Geometry check sheet. Reference: drawing and pictorial views, mm from the part's lowest x, y, z. A direction names the side the tool comes from. Round coordinates to 2 decimals unless told otherwise and drop trailing zeros. Write each loop counter-clockwise with the first axis right and the second up, starting at its lowest first coordinate (ties: lowest second). Pieces come first, ordered by that corner, then holes. Notation, with made-up numbers: (10.5, 41) -> (21.5, 41) arc R17 cw to (21.5, 66) -> close; hole circle Ø11 at (52.5, 24.25). An arc over 180 degrees is marked (long way). Write item = value, one per line.
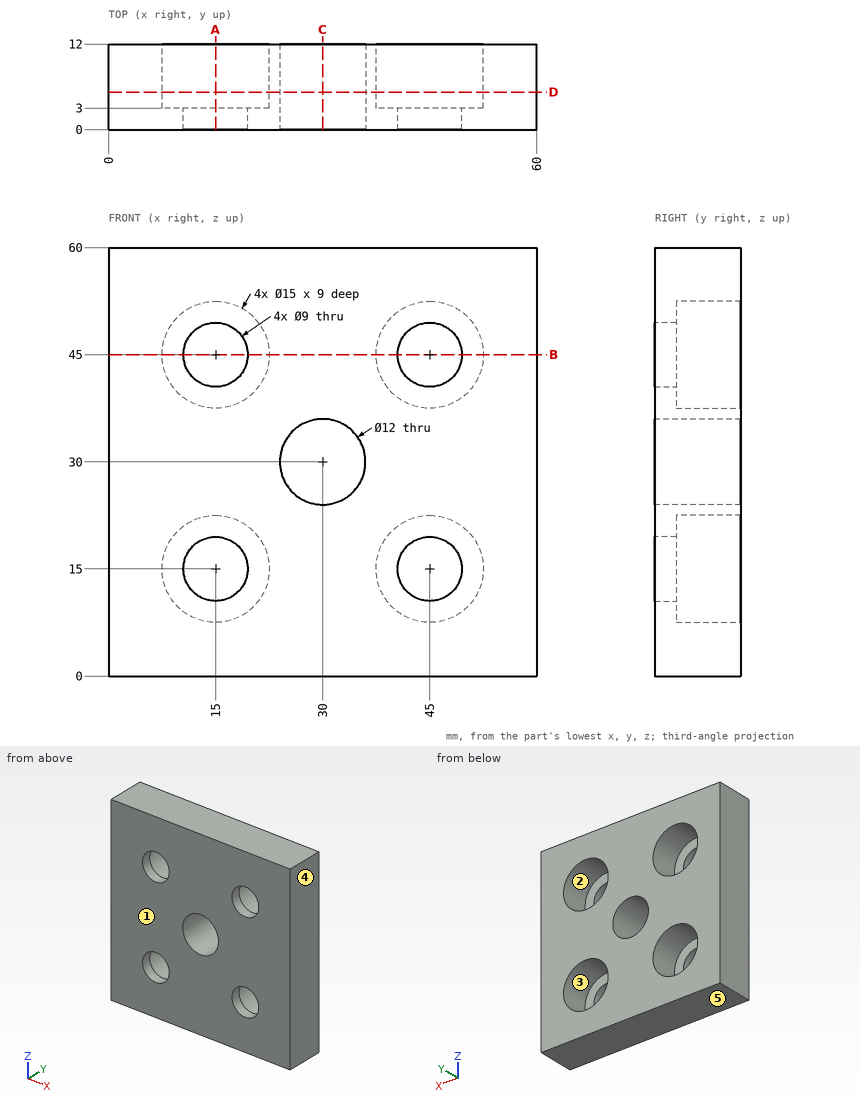
(1) Go/stop test with a flat-tipped pin: P1, Ø7.5, axis at x = 44, z = 48.5, coming from the +Y side. Record where the tip stops, or that it passes through.
Worked answers:
P1 = 3
(2) Sectioned sample at D-D on y = 5.25. Enter the section's corners in (x, z).
Worked answers:
outline = (0, 0) -> (60, 0) -> (60, 60) -> (0, 60) -> close; hole circle Ø15 at (15, 15); hole circle Ø15 at (15, 45); hole circle Ø12 at (30, 30); hole circle Ø15 at (45, 15); hole circle Ø15 at (45, 45)
(3) Sectioned sample at C-C on x = 30. Enter the section's corners in (y, z), then the cut area to 3 significant figures.
Worked answers:
outline = (0, 0) -> (12, 0) -> (12, 24) -> (0, 24) -> close; (0, 36) -> (12, 36) -> (12, 60) -> (0, 60) -> close
area = 576 mm²
(4) Release check for a two-part mould opening along Z. For the marked faces 3, 4 and 5 record: pulls with the +Z half, pulls with the -Z half, needs draft (parallel to the pull), parting line crosses it, or undercut.
Worked answers:
face_3 = undercut
face_4 = needs draft
face_5 = pulls with the -Z half
(5) Sectioned sample at B-B on z = 45. Enter the section's corners in (x, y).
Worked answers:
outline = (0, 0) -> (10.5, 0) -> (10.5, 3) -> (7.5, 3) -> (7.5, 12) -> (0, 12) -> close; (19.5, 0) -> (40.5, 0) -> (40.5, 3) -> (37.5, 3) -> (37.5, 12) -> (22.5, 12) -> (22.5, 3) -> (19.5, 3) -> close; (49.5, 0) -> (60, 0) -> (60, 12) -> (52.5, 12) -> (52.5, 3) -> (49.5, 3) -> close
(6) Material ranges on L1, parallel to X at y = 1.8, z = 15; L2, parallel to Z at x = 14.5, y = 7; L3, parallel to X at y = 8, z = 45, recorded low to high. Write a range as [from, to].
Worked answers:
L1 = [0, 10.5], [19.5, 40.5], [49.5, 60]
L2 = [0, 7.52], [22.48, 37.52], [52.48, 60]
L3 = [0, 7.5], [22.5, 37.5], [52.5, 60]
(7) Sectioned sample at A-A on x = 15. Enter the section's corners in (y, z), then the cut area to 3 significant figures.
Worked answers:
outline = (0, 0) -> (12, 0) -> (12, 7.5) -> (3, 7.5) -> (3, 10.5) -> (0, 10.5) -> close; (0, 19.5) -> (3, 19.5) -> (3, 22.5) -> (12, 22.5) -> (12, 37.5) -> (3, 37.5) -> (3, 40.5) -> (0, 40.5) -> close; (0, 49.5) -> (3, 49.5) -> (3, 52.5) -> (12, 52.5) -> (12, 60) -> (0, 60) -> close
area = 396 mm²
(8) Access from +Z, -Z, +X, -X, +Y, -Y to the whole of each face (thin tool, end or side, straight path). Record for the marked faces 1 and 2.
Worked answers:
face_1 = +Z, -Z, +X, -X, -Y
face_2 = +Y
